from build123d import *

# Parameters (mm, degrees)
CROQUIS1_R              = 11
SALIENTE_EXTRUIR1_DEPTH = 5
CROQUIS2_OUTSIDE_W      = 289.33
CROQUIS2_OUTSIDE_H      = 293.506
CROQUIS2_OUTSIDE_R      = 13.5
CORTAR_EXTRUIR1_DEPTH   = 22.219095174
CORTAR_EXTRUIR1_DRAFT   = -80
CROQUIS3_OUTSIDE_W      = 94.022
CROQUIS3_OUTSIDE_H      = 98.198
CROQUIS3_OUTSIDE_R      = 13.5
CORTAR_EXTRUIR2_DEPTH   = 5
CORTAR_EXTRUIR2_DRAFT   = -80


with BuildPart() as part:
    # Croquis1 → Saliente-Extruir1 (new body)
    with BuildSketch(Plane(origin=(0, 0, 0), x_dir=(1, 0, 0), z_dir=(0, 1, 0))):
        Polygon((0, 15.588457268), (-13.5, 7.794228634), (-13.5, -7.794228634), (0, -15.588457268), (13.5, -7.794228634), (13.5, 7.794228634), align=None)
        with Locations(Location((0, 0, 0), (0, 0, 270))):
            Circle(CROQUIS1_R, mode=Mode.SUBTRACT)
    extrude(amount=SALIENTE_EXTRUIR1_DEPTH)


with BuildPart() as cortar_extruir1_tool:
    # Croquis2 outside → Cortar-Extruir1 (with draft: the straight prism first)
    with BuildSketch(Plane(origin=(0, 5, 0), x_dir=(1, 0, 0), z_dir=(0, 1, 0))):
        Rectangle(CROQUIS2_OUTSIDE_W, CROQUIS2_OUTSIDE_H)
        Circle(CROQUIS2_OUTSIDE_R, mode=Mode.SUBTRACT)
    extrude(amount=-CORTAR_EXTRUIR1_DEPTH)
    # Cortar-Extruir1: the draft: its side faces are tilted about the plane it starts from
    cortar_extruir1_sides = [cortar_extruir1_tool.faces().sort_by_distance(p)[0] for p in [
        (0, -6.109547587, 146.753),
        (144.665, -6.109547587, 0),
        (0, -6.109547587, -146.753),
        (-144.665, -6.109547587, 0),
        (-13.5, -6.109547587, 0),
    ]]
    draft(cortar_extruir1_sides, Plane(origin=(0, 5, 0), x_dir=(1, 0, 0), z_dir=(0, 1, 0)), CORTAR_EXTRUIR1_DRAFT)


with BuildPart() as part_1:
    add(part.part)

    # Cortar-Extruir1: cut by cortar_extruir1_tool
    add(cortar_extruir1_tool.part, mode=Mode.SUBTRACT)


with BuildPart() as cortar_extruir2_tool:
    # Croquis3 outside → Cortar-Extruir2 (with draft: the straight prism first)
    with BuildSketch(Plane.XZ):
        Rectangle(CROQUIS3_OUTSIDE_W, CROQUIS3_OUTSIDE_H)
        Circle(CROQUIS3_OUTSIDE_R, mode=Mode.SUBTRACT)
    extrude(amount=-CORTAR_EXTRUIR2_DEPTH)
    # Cortar-Extruir2: the draft: its side faces are tilted about the plane it starts from
    cortar_extruir2_sides = [cortar_extruir2_tool.faces().sort_by_distance(p)[0] for p in [
        (0, 2.5, -49.099),
        (47.011, 2.5, 0),
        (0, 2.5, 49.099),
        (-47.011, 2.5, 0),
        (-13.5, 2.5, 0),
    ]]
    draft(cortar_extruir2_sides, Plane.XZ, CORTAR_EXTRUIR2_DRAFT)


with BuildPart() as part_2:
    add(part_1.part)

    # Cortar-Extruir2: cut by cortar_extruir2_tool
    add(cortar_extruir2_tool.part, mode=Mode.SUBTRACT)


solid = part_2.part
Could you check a few things on this model? Use its own coordinates, in mm. Coordinates: 2 decimals unless noted, no trailing zeros. Loops run counter-clockwise (first coordinate to the right, second up) from the corner with the lowest first, then second, coordinate; pieces in that order, holes last.
1. Imagine slicing it at A-A (y = 3.35). Please give me the cut outline in (x, z).
2. For P1, Ø3, axis at y = 2, z = -9.5, coming from the +X side, with a flat end and sliding along its axis, tell me the tip position at first contact or that it passes through.
3. We'd pull the mould along Y, two halves only. Please class faces 1 (the face through (-12.11, 4.91, -7.03)), 2 (the face through (0.03, 0.09, 14)), 3 (the face through (-6.84, 2.46, 11.64)): released by +Y, released by -Y, zero draft, split by the parting line, or undercut.
4. I need wall thicknesses on L1, parallel to X at y = 2.35, z = 0; L2, parallel to Z at x = -3, y = 3.4; L3, parallel to Z at x = 6.5, y = 2.15. Which ranges of each line are inside material? Lowest first, please.
Computed values:
1. outline: (-13.5, -7.79) - (0, -15.59) - (13.5, -7.79) - (13.5, 7.79) - (0, 15.59) - (-13.5, 7.79) - close; hole circle Ø22 at (0, 0)
2. P1: stops at x = 13.14
3. face 1: released by +Y
3. face 2: released by -Y
3. face 3: zero draft
4. L1: x = -13.5 to -11, 11 to 13.5
4. L2: z = -13.86 to -10.58, 10.58 to 13.86
4. L3: z = -11.84 to -8.87, 8.87 to 11.84
